Could you check a few things on this model? Use its own coordinates, in mm. Face numbers are marked on the shaded views. A direction names the side the tool comes from. Round coordinates to 2 decimals unless told otherwise and drop trailing zeros. Order: outer loops, then holes, each group sorted by start corner. A loop starts at its lowest first (then second) coordinate and runs counter-clockwise, first axis right, second up. Notation, with made-up numbers: (70, 48.25) -> (99, 48.25) arc R17 cw to (99, 71.25) -> close; hole circle Ø1 at (-31.75, 62). An arc over 180 degrees is marked (long way). One line per question, with ' | ' between items.
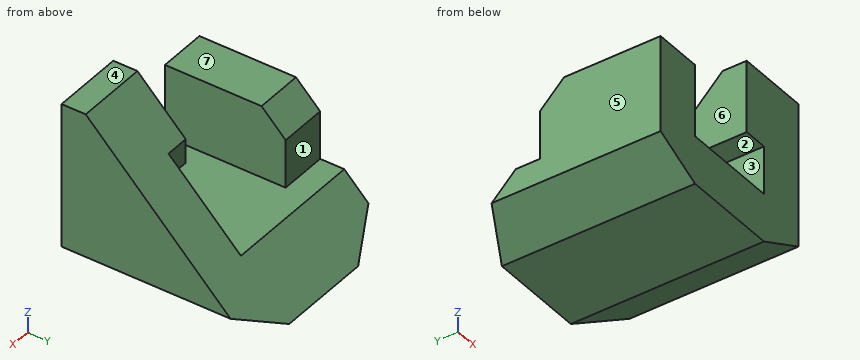
```python
from build123d import *

# Parameters (mm, degrees)
SKETCH1_W           = 40
SKETCH1_H           = 40
BOSS_EXTRUDE1_DEPTH = 35
CUT_EXTRUDE1_DEPTH  = 41
CUT_EXTRUDE3_DEPTH  = 41
CUT_EXTRUDE4_DEPTH  = 5
SKETCH5_W           = 10
SKETCH5_H           = 25
BOSS_EXTRUDE2_DEPTH = 15
CUT_EXTRUDE5_DEPTH  = 15
CUT_EXTRUDE6_DEPTH  = 41


with BuildPart() as part:
    # Sketch1 → Boss-Extrude1 (new body)
    with BuildSketch(Plane.XY):
        Rectangle(SKETCH1_W, SKETCH1_H)
    extrude(amount=BOSS_EXTRUDE1_DEPTH)

    # Sketch2 → Cut-Extrude1 (cut, through all)
    with BuildSketch(Plane(origin=(0, 20, 0), x_dir=(1, 0, 0), z_dir=(0, 1, 0))):
        Polygon((-20, -10), (10, -10), (10, -20), (5, -20), (5, -35), (-20, -35), align=None)
    extrude(amount=-CUT_EXTRUDE1_DEPTH, mode=Mode.SUBTRACT)

    # Sketch3 → Cut-Extrude3 (cut, through all)
    with BuildSketch(Plane(origin=(-20, 0, 0), x_dir=(0, 0, -1), z_dir=(1, 0, 0))):
        Polygon((0, 20), (-35, -15), (-35, 20), align=None)
    extrude(amount=CUT_EXTRUDE3_DEPTH, mode=Mode.SUBTRACT)

    # Sketch4 → Cut-Extrude4 (cut)
    with BuildSketch(Plane.ZY.offset(-5)):
        Polygon((20, 0), (20, -5), (25, -5), align=None)
    extrude(amount=-CUT_EXTRUDE4_DEPTH, mode=Mode.SUBTRACT)

    # Sketch5 → Boss-Extrude2 (add)
    with BuildSketch(Plane.XY.offset(10)):
        with Locations((-15, -7.5)):
            Rectangle(SKETCH5_W, SKETCH5_H)
    extrude(amount=BOSS_EXTRUDE2_DEPTH)

    # Sketch6 → Cut-Extrude5 (cut)
    with BuildSketch(Plane.ZY.offset(20)):
        Polygon((25, 5), (20, 5), (25, 0), align=None)
    extrude(amount=-CUT_EXTRUDE5_DEPTH, mode=Mode.SUBTRACT)

    # Sketch7 → Cut-Extrude6 (cut, through all)
    with BuildSketch(Plane.XZ.offset(20)):
        Polygon((10, 0), (20, 5), (20, 0), align=None)
        Polygon((-20, 0), (-10, 0), (-20, 5), align=None)
    extrude(amount=-CUT_EXTRUDE6_DEPTH, mode=Mode.SUBTRACT)


solid = part.part
```
1. I need wall thicknesses on probe 1 along X at (y, z) = (-13, 23.5); probe 2 along X at (y, z) = (0, 17); probe 3 along X at (y, z) = (-2, 23.5). Which ranges of each line are inside material? Lowest first, please.
From the geometry:
probe 1: x = -20 to -10, 5 to 20 | probe 2: x = -20 to -10, 10 to 20 | probe 3: x = -20 to -10
2. I want a section at A-A on z = 23. List the corners of the cut face in (x, y) for me, and give its area (3 significant figures).
From the geometry:
outline: (-20, -20) -> (-10, -20) -> (-10, 2) -> (-20, 2) -> close; (5, -20) -> (20, -20) -> (20, -3) -> (10, -3) -> (10, -5) -> (5, -5) -> close | area: 465 mm²
3. I want a section at D-D on y = 8.5. List the corners of the cut face in (x, z) for me.
From the geometry:
outline: (-20, 5) -> (-10, 0) -> (10, 0) -> (20, 5) -> (20, 11.5) -> (10, 11.5) -> (10, 10) -> (-20, 10) -> close
4. On a 3-axis mill with a long thin cutter (end or side, diameter ignored), from which of +Z, -Z, +X, -X, +Y, -Y can I reach the whole of each face in a straight line? I mean the marked faces 5, 6 and 7. Say none if no direction works.
From the geometry:
face 5: +Z, -Z, -X, +Y, -Y | face 6: +Z, +Y, -Y | face 7: +Z, -X, +Y, -Y
5. I want a section at B-B on x = 7. List the corners of the cut face in (y, z) for me, and give its area (3 significant figures).
From the geometry:
outline: (-20, 0) -> (20, 0) -> (10, 10) -> (-20, 10) -> close; (-20, 20) -> (-5, 20) -> (-5, 25) -> (-15, 35) -> (-20, 35) -> close | area: 525 mm²
6. I want a section at C-C on y = -12. List the corners of the cut face in (x, z) for me, and give its area (3 significant figures).
From the geometry:
outline: (-20, 5) -> (-10, 0) -> (10, 0) -> (20, 5) -> (20, 32) -> (5, 32) -> (5, 20) -> (10, 20) -> (10, 10) -> (-10, 10) -> (-10, 25) -> (-20, 25) -> close | area: 780 mm²
7. If we mould it in two halves opening along Z, with no side actions, what happens to the marked faces 1, 2, 3 and 4? For each: pulls with the +Z half, pulls with the -Z half, needs draft (parallel to the pull), parting line crosses it, or undercut.
From the geometry:
face 1: needs draft | face 2: undercut | face 3: undercut | face 4: pulls with the +Z half
8. I'm going to push flat-ended pins straight in: pin 1 (5 mm diameter, centred on x = -0.5, y = 15, fed in from +Z); pin 2 (3 mm diameter, centred on x = -14.5, z = 17, fed in from +Y); pin 3 (15 mm diameter, centred on x = -11, y = -8.5, fed in from +Z). Where does each tip first touch, or does it pass through?
From the geometry:
pin 1: stops at z = 7.5 | pin 2: stops at y = 5 | pin 3: stops at z = 25
